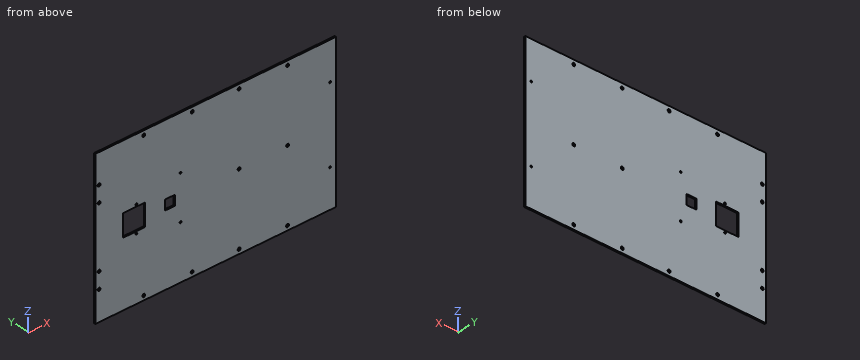
from build123d import *

# Parameters (mm, degrees)
SKETCH1_W                    = 199.39
SKETCH1_H                    = 127
BOSS_EXTRUDE1_DEPTH          = 2.54
F_11_0_191_DIAMETER_HOLE1_D  = 4.8514
F_11_0_191_DIAMETER_HOLE2_D  = 4.8514
SKETCH8_W                    = 36.83
SKETCH8_H                    = 18.415
SKETCH8_W_2                  = 16.51
SKETCH8_H_2                  = 8.255
CUT_EXTRUDE1_DEPTH           = 2.54
F_11_0_191_DIAMETER_HOLE3_D  = 4.8514
F_31_0_12_DIAMETER_HOLE2_D   = 3.048
F_31_0_12_DIAMETER_HOLE3_D   = 3.048
F_1_8_0_125_DIAMETER_HOLE1_D = 3.048


with BuildPart() as part:
    # Sketch1 → Boss-Extrude1 (new body)
    with BuildSketch(Plane(origin=(0, 0, 0), x_dir=(1, 0, 0), z_dir=(0, 1, 0))):
        with Locations((-99.695, 0)):
            Rectangle(SKETCH1_W, SKETCH1_H)
        with Locations((99.695, 0)):
            Rectangle(SKETCH1_W, SKETCH1_H)
    boss_extrude1 = extrude(amount=BOSS_EXTRUDE1_DEPTH)

    # #11 (0.191) Diameter Hole1 (through all)
    with Locations(Plane(origin=(0, 2.54, 0), x_dir=(1, 0, 0), z_dir=(0, 1, 0))):
        with Locations((-193.167, -14.4018), (-193.04, 12.3444)):
            f_11_0_191_diameter_hole1 = Hole(F_11_0_191_DIAMETER_HOLE1_D / 2)

    # #11 (0.191) Diameter Hole2 (through all)
    with Locations(Plane(origin=(0, 2.54, 0), x_dir=(1, 0, 0), z_dir=(0, 1, 0))):
        with Locations((-119.126, -56.127777467), (-38.862, -56.127777467), (38.862, -56.127777467), (119.126, -56.127777467)):
            f_11_0_191_diameter_hole2 = Hole(F_11_0_191_DIAMETER_HOLE2_D / 2)

    # Sketch8 → Cut-Extrude1 (cut)
    with BuildSketch(Plane(origin=(0, 2.54, 0), x_dir=(1, 0, 0), z_dir=(0, 1, 0))):
        with Locations((-135.255, 54.2925)):
            Rectangle(SKETCH8_W, SKETCH8_H)
        with Locations((-75.565, 59.3725)):
            Rectangle(SKETCH8_W_2, SKETCH8_H_2)
    cut_extrude1 = extrude(amount=-CUT_EXTRUDE1_DEPTH, mode=Mode.SUBTRACT)

    # Mirror6: Boss-Extrude1, #11 (0.191) Diameter Hole1, #11 (0.191) Diameter Hole2, Cut-Extrude1 across plane
    add(boss_extrude1.mirror(Plane(origin=(0, 2.54, -63.5), x_dir=(1, 0, 0), z_dir=(0, 0, -1))))
    add(f_11_0_191_diameter_hole1.mirror(Plane(origin=(0, 2.54, -63.5), x_dir=(1, 0, 0), z_dir=(0, 0, -1))), mode=Mode.SUBTRACT)
    add(f_11_0_191_diameter_hole2.mirror(Plane(origin=(0, 2.54, -63.5), x_dir=(1, 0, 0), z_dir=(0, 0, -1))), mode=Mode.SUBTRACT)
    add(cut_extrude1.mirror(Plane(origin=(0, 2.54, -63.5), x_dir=(1, 0, 0), z_dir=(0, 0, -1))), mode=Mode.SUBTRACT)

    # #11 (0.191) Diameter Hole3 (through all)
    with Locations(Plane(origin=(0, 2.54, 0), x_dir=(1, 0, 0), z_dir=(0, 1, 0))):
        with Locations((119.126, 63.5), (38.862, 63.5)):
            Hole(F_11_0_191_DIAMETER_HOLE3_D / 2)

    # #31 (0.12) Diameter Hole2 (through all)
    with Locations(Plane(origin=(0, 2.54, 0), x_dir=(1, 0, 0), z_dir=(0, 1, 0))):
        with Locations((-131.318, 41.656), (-131.318, 85.344)):
            Hole(F_31_0_12_DIAMETER_HOLE2_D / 2)

    # #31 (0.12) Diameter Hole3 (through all)
    with Locations(Plane(origin=(0, 2.54, 0), x_dir=(1, 0, 0), z_dir=(0, 1, 0))):
        with Locations((-58.166, 100.33), (-58.166, 26.67)):
            Hole(F_31_0_12_DIAMETER_HOLE3_D / 2)

    # 1/8 (0.125) Diameter Hole1 (through all)
    with Locations(Plane(origin=(0, 2.54, 0), x_dir=(1, 0, 0), z_dir=(0, 1, 0))):
        with Locations((189.484, 0), (189.484, 127)):
            Hole(F_1_8_0_125_DIAMETER_HOLE1_D / 2)


solid = part.part
Model file for the job. Use its own axes, mm. Coordinates: 2 decimals unless noted, no trailing zeros. One line per item, written item: value. Start each with the question number.
1) Flat gauge pins, fed straight in: pin 1 Ø3 at (x, z) = (-119.13, -183.13) entering from +Y; pin 2 Ø8 at (x, z) = (-193.17, 14.4) entering from +Y. Where does each tip first touch, or does it go through?
2) Probe probe 1 along X at (y, z) = (1.5, -69.5); probe 2 along Z at (x, y) = (-79, 0.9) (3 decimals); probe 3 along Z at (x, y) = (-149.5, 2) (3 decimals). List the from-to ranges inside material, lowest first.
3) Slice it at A-A on y = 0.6. Count the separate pieces of the cut face and the enclosed holes in it, then the cut area to 3 significant figures.
Answers follow:
1. pin 1: through
1. pin 2: y = 2.54
2. probe 1: -199.39 to -153.67, -116.84 to -83.82, -67.31 to 199.39
2. probe 2: -190.5 to -71.755, -55.245 to 63.5
2. probe 3: -190.5 to -81.915, -45.085 to 63.5
3. separate pieces: 1
3. enclosed holes: 22
3. area: 99,400 mm2
